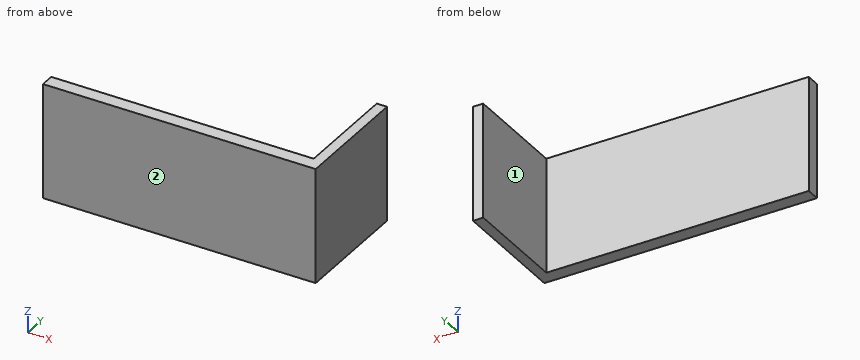
from build123d import *

# Parameters (mm, degrees)
F2_DEPTH = 76.2
F3_DEPTH = 76.2


# Not quite as in the source:
# - the program builds the solid bodies; features that only make, move or delete a surface that nothing else refers to are left out


with BuildPart() as f2:
    # F0 (on Top) → F2 (new body)
    with BuildSketch(Plane.XY):
        Polygon((88.587783277, 43.1846939027), (81.7847177386, 43.1846939027), (81.7847177386, -26.9164871424), (-92.4329981208, -26.9164871424), (-92.4329981208, -36.0858403146), (88.587783277, -36.0858403146), align=None)
    extrude(amount=F2_DEPTH)

    # F0 (on Top) → F3 (join)
    with BuildSketch(Plane.XY):
        Polygon((88.587783277, 43.1846939027), (81.7847177386, 43.1846939027), (81.7847177386, -26.9164871424), (-92.4329981208, -26.9164871424), (-92.4329981208, -36.0858403146), (88.587783277, -36.0858403146), align=None)
    extrude(amount=F3_DEPTH)


solid = f2.part
Can you work these out from the model? Positions are in its coordinate system, mm. Face numbers are marked on the shaded views. A direction names the side the tool comes from. Round coordinates to 2 decimals unless told otherwise and drop trailing zeros. Write each loop counter-clockwise with the first axis right and the second up, starting at its lowest first coordinate (ties: lowest second). Pieces come first, ordered by that corner, then holes. Notation, with made-up numbers: (56.5, 12) -> (105.5, 12) arc R17 ccw to (105.5, 19) -> close; hole circle Ø6 at (18, 25). An arc over 180 degrees is marked (long way). Use one line per item in the form item = value. Start each with the question number.
Q1. I'm going to push flat-ended pins straight in: P1, Ø1, axis at y = 3.5, z = 19.5, coming from the -X side; P2, Ø12, axis at x = 68, z = 41, coming from the +Y side. Where does each tip first touch, or does it pass through?
Q2. If I drill on probe 1 along X at (y, z) = (29, 71); probe 2 along Y at (x, z) = (-18, 40), over which ranges is the centre line in solid material (lowest first)? Write a range as [from, to].
Q3. Which directions (+Z, -Z, +X, -X, +Y, -Y) give clear straight access to the entire face, cutting with the end or side of a thin tool? Please do the marked faces 1 and 2.
Q4. Imagine slicing it at A-A (z = 70). Please give me the cut outline in (x, y), then the cut area to 3 significant figures.
Q5. Imagine slicing it at B-B (y = 31). Please give me the cut outline in (x, z), then the cut area to 3 significant figures.
Q6. Imagine slicing it at C-C (x = -79). Please give me the cut outline in (y, z), then the cut area to 3 significant figures.
Worked out:
q1.P1 = 81.78
q1.P2 = -26.92
q2.probe_1 = [81.78, 88.59]
q2.probe_2 = [-36.09, -26.92]
q3.face_1 = +Z, -Z, -X, +Y
q3.face_2 = +Z, -Z, +X, -X, -Y
q4.outline = (-92.43, -36.09) -> (88.59, -36.09) -> (88.59, 43.18) -> (81.78, 43.18) -> (81.78, -26.92) -> (-92.43, -26.92) -> close
q4.area = 2,140 mm^2
q5.outline = (81.78, 0) -> (88.59, 0) -> (88.59, 76.2) -> (81.78, 76.2) -> close
q5.area = 518 mm^2
q6.outline = (-36.09, 0) -> (-26.92, 0) -> (-26.92, 76.2) -> (-36.09, 76.2) -> close
q6.area = 699 mm^2
